Can you work these out from the drawing? Everything is in mm from the part's minimum corner. A direction names the side the tool comes from. Round coordinates to 2 decimals unless told otherwise and drop trailing zeros. Write each loop counter-clockwise with the first axis right and the second up, starting at its lowest first coordinate (ties: lowest second). Pieces come first, ordered by that corner, then holes. Notation, with made-up numbers: (27, 72) - (82, 72) arc R29 cw to (82, 102) - close; hole circle Ø3 at (8.5, 83). An arc over 180 degrees is marked (long way). Write each question's results on one line, items separated by ' | '. Start each with the question number.
(1) Please list where these lines run through material, in increasing order: line 1 (X direction, y = 43, z = 19); line 2 (Y direction, x = 36, z = 18.75); line 3 (X direction, y = 69.5, z = 1.75). Write a range as [from, to].
(2) On a 3-axis mill with a long thin cutter (end or side, diameter ignored), from which of +Z, -Z, +X, -X, +Y, -Y can I reach the whole of each face in a straight line? I mean the marked faces 1, 2 and 3. Say none if no direction works.
(3) Imagine slicing it at C-C on x = 51. Write out the boundary of the cut face in (y, z) (3 decimals), then the cut area to 3 significant figures.
(4) For P1, Ø5.5, axis at y = 63, z = 10.5, coming from the +X side; P2, Ø1.5, axis at x = 10, z = 10.5, coming from the +Y side; P3, Ø8, axis at x = 26.5, y = 75, coming from the +Z side, each with a flat end and sliding along its axis, tell me the tip position at first contact or that it passes through.
(5) Imagine slicing it at D-D on z = 8.75. Write out the boundary of the cut face in (x, y), then the cut area to 3 significant figures.
(6) Imagine slicing it at A-A on z = 17.25. Write out the boundary of the cut face in (x, y), then the cut area to 3 significant figures.
(7) Thinking about a two-plate mould opening in Y: for the marked faces 4, 5 and 6, which applies, +Y half, -Y half, draft (parallel to the pull), parting line (faces both ways), or undercut?
(8) Imagine slicing it at B-B on y = 50. Write out the boundary of the cut face in (x, z).
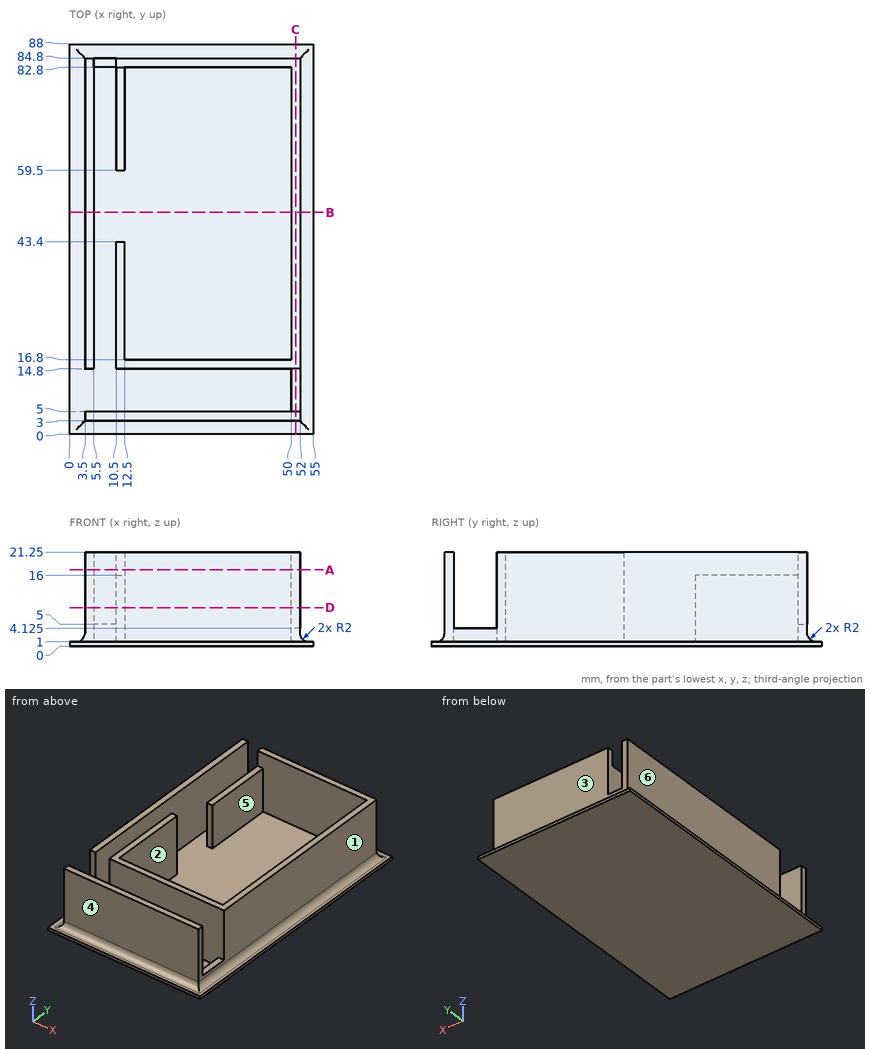
Response:
1) line 1: [3.5, 5.5], [10.5, 12.5], [50, 52] | line 2: [3, 5], [14.8, 16.8], [82.8, 84.8] | line 3: [3.06, 5.5], [10.5, 12.5], [50, 52.44]
2) face 1: +Z, +X, +Y, -Y | face 2: +Z | face 3: +Z, +X, -X, +Y
3) outline: (0, 0) - (88, 0) - (88, 1) - (86.8, 1) arc R2 cw to (84.8, 3) - (84.8, 21.25) - (14.8, 21.25) - (14.8, 4.125) - (5, 4.125) - (5, 21.25) - (3, 21.25) - (3, 3) arc R2 cw to (1, 1) - (0, 1) - close | area: 1,580 mm²
4) P1: x = 52 | P2: y = 84.8 | P3: z = 1
5) outline: (3.5, 3) - (52, 3) - (52, 5) - (3.5, 5) - close; (3.5, 14.8) - (5.5, 14.8) - (5.5, 84.8) - (3.5, 84.8) - close; (10.5, 14.8) - (52, 14.8) - (52, 84.8) - (10.5, 84.8) - (10.5, 59.5) - (12.5, 59.5) - (12.5, 82.8) - (50, 82.8) - (50, 16.8) - (12.5, 16.8) - (12.5, 43.4) - (10.5, 43.4) - close | area: 635 mm²
6) outline: (3.5, 3) - (52, 3) - (52, 5) - (3.5, 5) - close; (3.5, 14.8) - (5.5, 14.8) - (5.5, 84.8) - (3.5, 84.8) - close; (10.5, 14.8) - (52, 14.8) - (52, 84.8) - (10.5, 84.8) - (10.5, 82.8) - (50, 82.8) - (50, 16.8) - (12.5, 16.8) - (12.5, 43.4) - (10.5, 43.4) - close | area: 588 mm²
7) face 4: -Y half | face 5: undercut | face 6: draft
8) outline: (0, 0) - (55, 0) - (55, 1) - (54, 1) arc R2 cw to (52, 3) - (52, 21.25) - (50, 21.25) - (50, 1) - (5.5, 1) - (5.5, 21.25) - (3.5, 21.25) - (3.5, 3) arc R2 cw to (1.5, 1) - (0, 1) - close
